from build123d import *

# Parameters (mm, degrees)
SKETCH1_W           = 120
SKETCH1_H           = 180
BOSS_EXTRUDE1_DEPTH = 10
SKETCH2_R           = 4
SKETCH2_R_2         = 1.5
CUT_EXTRUDE1_DEPTH  = 10
SKETCH3_W           = 67
SKETCH3_H           = 54
SKETCH3_W_2         = 85
SKETCH3_H_2         = 41
SKETCH3_W_3         = 10.36
SKETCH3_H_3         = 14.7
CUT_EXTRUDE2_DEPTH  = 2
SKETCH4_W           = 8.5
SKETCH4_H           = 13
CUT_EXTRUDE3_DEPTH  = 10


with BuildPart() as part:
    # Sketch1 → Boss-Extrude1 (new body)
    with BuildSketch(Plane(origin=(0, 0, 0), x_dir=(1, 0, 0), z_dir=(0, 1, 0))):
        with Locations((-19.57251684, 15.427483158)):
            Rectangle(SKETCH1_W, SKETCH1_H)
    extrude(amount=BOSS_EXTRUDE1_DEPTH)

    # Sketch2 → Cut-Extrude1 (cut)
    with BuildSketch(Plane.XZ):
        with Locations(Location((-73.57251684, 50.65020927, 0), (0, 0, 270))):
            Circle(SKETCH2_R)
        with Locations(Location((34.42748316, 50.65020927, 0), (0, 0, 270))):
            Circle(SKETCH2_R)
        with Locations(Location((34.42748316, -81.427483158, 0), (0, 0, 270))):
            Circle(SKETCH2_R)
        with Locations(Location((-73.57251684, -81.427483158, 0), (0, 0, 270))):
            Circle(SKETCH2_R)
        with Locations(Location((-73.57251684, -9.34979073, 0), (0, 0, 270))):
            Circle(SKETCH2_R_2)
        with Locations(Location((34.42748316, -9.34979073, 0), (0, 0, 270))):
            Circle(SKETCH2_R_2)
    extrude(amount=-CUT_EXTRUDE1_DEPTH, mode=Mode.SUBTRACT)

    # Sketch3 → Cut-Extrude2 (cut)
    with BuildSketch(Plane.XZ):
        with Locations((-20.178258513, 45.076374251)):
            Rectangle(SKETCH3_W, SKETCH3_H)
        with Locations((-14.626073682, -76.328520248)):
            Rectangle(SKETCH3_W_2, SKETCH3_H_2)
        with Locations((-71.569507279, -63.427483158)):
            Rectangle(SKETCH3_W_3, SKETCH3_H_3)
    extrude(amount=-CUT_EXTRUDE2_DEPTH, mode=Mode.SUBTRACT)

    # Sketch4 → Cut-Extrude3 (cut)
    with BuildSketch(Plane.XZ):
        with Locations((-71.569507279, -63.427483158)):
            Rectangle(SKETCH4_W, SKETCH4_H)
    extrude(amount=-CUT_EXTRUDE3_DEPTH, mode=Mode.SUBTRACT)


solid = part.part
Design review of the part built by this model. Coordinates are the model's own, in mm. A direction names the side the tool comes from. Give positions to 0.01 mm unless a question says otherwise; leave off trailing zeros. Loops run counter-clockwise (first coordinate to the right, second up) from the corner with the lowest first, then second, coordinate; pieces in that order, holes last. Notation, with made-up numbers: (18, -28.75) -> (25, -28.75) arc R32 cw to (25, -2.75) -> close; hole circle Ø9 at (-26, 85). An arc over 180 degrees is marked (long way). One line per question, with ' | ' between items. Start each with the question number.
(1) We need section B-B (x = 8). State the section outline as (y, z) points.
(2) For line 1 (X direction, y = 2.5, z = 51); line 2 (Z direction, x = 16.5, y = 1.75); line 3 (Z direction, x = -74, y = 8), list the stretches that pass through material, from the lowest coordinate up.
(3) We need section C-C (z = 40.5). State the section outline as (x, y) points, and give its area (3 significant figures).
(4) For faces 1 (the face through (-79.573, 5, -14)), 2 (the face through (-76, 2, -63)), 3 (the face through (-72, 6, -69.927)), list the 3-axis set-ups (+Z, -Z, +X, -X, +Y, -Y) from which the entire face can be reached by the end or side of a thin tool; tool diameter is ignored.
(5) We need section D-D (y = 4). State the section outline as (x, z) points.
(6) Insertion check: P1, Ø20.5, axis at x = -6, z = -69.5, coming from the -Y side. The pin has a flat end and moves straight along its axis. Give the tip position at first contact, or say it passes through.
(7) Draft analysis for pull direction Z (two halves, no side actions). For faces 4 (the face through (-72, 6, -56.927)), 5 (the face through (-20, 10, -17)), 6 (the face through (-20, 5, 74.573)), 7 (the face through (-76.006, 4.93, -78.253)), state which applies: +Z half, -Z half, draft (parallel to the pull), parting line (faces both ways), or undercut.
(8) We need section A-A (z = -67). State the section outline as (x, y) points.
The answers:
1) outline: (0, -105.43) -> (10, -105.43) -> (10, 74.57) -> (0, 74.57) -> (0, 72.08) -> (2, 72.08) -> (2, 18.08) -> (0, 18.08) -> (0, -55.83) -> (2, -55.83) -> (2, -96.83) -> (0, -96.83) -> close
2) line 1: x = -79.57 to -77.56, -69.59 to 30.44, 38.41 to 40.43 | line 2: z = -105.43 to -96.83, -55.83 to 74.57 | line 3: z = -105.43 to -85.4, -77.45 to -69.93, -56.93 to -10.79, -7.91 to 46.67, 54.63 to 74.57
3) outline: (-79.57, 0) -> (-53.68, 0) -> (-53.68, 2) -> (13.32, 2) -> (13.32, 0) -> (40.43, 0) -> (40.43, 10) -> (-79.57, 10) -> close | area: 1,070 mm^2
4) face 1: +Z, -Z, -X, +Y, -Y | face 2: -Y | face 3: +Y, -Y
5) outline: (-79.57, -105.43) -> (40.43, -105.43) -> (40.43, 74.57) -> (-79.57, 74.57) -> close; hole circle Ø8 at (-73.57, -81.43); hole circle Ø8 at (-73.57, 50.65); hole (-75.82, -69.93) -> (-67.32, -69.93) -> (-67.32, -56.93) -> (-75.82, -56.93) -> close; hole circle Ø3 at (-73.57, -9.35); hole circle Ø8 at (34.43, -81.43); hole circle Ø8 at (34.43, 50.65); hole circle Ø3 at (34.43, -9.35)
6) P1: stops at y = 2
7) face 4: undercut | face 5: draft | face 6: +Z half | face 7: undercut
8) outline: (-79.57, 0) -> (-76.75, 0) -> (-76.75, 2) -> (-75.82, 2) -> (-75.82, 10) -> (-79.57, 10) -> close; (-67.32, 2) -> (-66.39, 2) -> (-66.39, 0) -> (-57.13, 0) -> (-57.13, 2) -> (27.87, 2) -> (27.87, 0) -> (40.43, 0) -> (40.43, 10) -> (-67.32, 10) -> close
